Source: CAD feature listing. Evaluate the final solid. Frame: model axes, mm. A direction names the side the tool comes from. Round coordinates to 2 decimals unless told otherwise and drop trailing zeros. Loops run counter-clockwise (first coordinate to the right, second up) from the corner with the lowest first, then second, coordinate; pieces in that order, holes last.
(1) Material intervals for probe 1 along X at (y, z) = (0, 5); probe 2 along X at (y, z) = (16, 2) (3 decimals); probe 3 along Z at (x, y) = (11.25, -2), sorted ascending.
(2) First-contact query: pin 1 Ø5.5 at (x, y) = (7.94, 0) entering from +Z (3 decimals); pin 2 Ø5 at (y, z) = (-10.1, 10.1) entering from -X; pin 3 Ø2 at (x, y) = (2, 13) entering from +Z; pin 4 Ø6 at (x, y) = (1.5, 14.5) entering from +Z. Flat tips, straight axial feed; report the tip coordinate or a pass-through.
(3) Section D-D, the plane z = 5. Return the cut outline in (x, y) (1 decimal), plus the area to 3 significant figures.
(4) Section B-B, the plane x = 2. Return the cut outline in (y, z).
(5) Section A-A, the plane z = 11. Return the cut outline in (x, y) (3 decimals), plus the area to 3 significant figures.
(6) Mould query, pull axis Z, two halves, no side actions, for faces 3 (the cylindrical face through (1.565, -8.319, 8.735)), 4 (the cylindrical face through (9.663, 0.076, 6.049)), 5 (the cylindrical face through (1.565, 11.887, 8.735)), 6 (the cylindrical face through (7.87, -2.06, -9.3)). Classes: pulls with the +Z half, pulls with the -Z half, needs draft (parallel to the pull), parting line crosses it, or undercut.
(7) Section C-C, the plane y = -4. Return the cut outline in (x, z) (3 decimals).
(8) Set-up query: faces 1 (the cylindrical face through (1.57, -15.12, -11.59)), 2 (the flat face through (3.175, 4, 9)). Return all of +Z, -Z, +X, -X, +Y, -Y with unobstructed straight access to the full face (end or side cutting, diameter ignored); none if empty.
```python
from build123d import *

# Parameters (mm, degrees)
F0_R     = 19.05
F1_DEPTH = 3.175
F2_R     = 9.525
F3_DEPTH = 9.525
F5_D     = 6.35
F5_DEPTH = 9.525
F5_TIP   = 1.9077324654
F8_D     = 3.4544
F8_DEPTH = 9.525
F8_START = 0.1579085
F8_TIP   = 1.0378064612
F10_D    = 4.4958


with BuildPart() as f1:
    # F0 (on Right) → F1 (new body)
    with BuildSketch(Plane.YZ):
        Circle(F0_R)
    extrude(amount=F1_DEPTH)

    # F2 (on face) → F3 (join)
    with BuildSketch(Plane.YZ.offset(3.175)):
        Circle(F2_R)
    extrude(amount=F3_DEPTH)

    # F5
    with Locations(Plane.YZ.offset(12.7)):
        with Locations((0, 0)):
            Hole(F5_D / 2, depth=F5_DEPTH)
            with Locations((0, 0, -(F5_DEPTH + F5_TIP / 2))):  # 118° drill point
                Cone(0, F5_D / 2, F5_TIP, mode=Mode.SUBTRACT)

    # F8
    # its depths count from where the whole tool has entered the part; down to there all is cleared
    with Locations(Plane.XY.offset(9.525).offset(-F8_START)):
        with Locations((7.9375, 0)):
            Hole(F8_D / 2, depth=F8_DEPTH)
            with Locations((0, 0, -(F8_DEPTH + F8_TIP / 2))):  # 118° drill point
                Cone(0, F8_D / 2, F8_TIP, mode=Mode.SUBTRACT)

    # F10 (through all)
    with Locations(Plane.YZ.offset(3.175)):
        with Locations((-10.1027881362, 10.1027881362), (10.1027881362, 10.1027881362), (10.1027881362, -10.1027881362), (-10.1027881362, -10.1027881362)):
            Hole(F10_D / 2)


solid = f1.part
```
Output values:
1. probe 1: x = 0 to 6.21, 9.66 to 12.7
1. probe 2: x = 0 to 3.175
1. probe 3: z = -9.31 to -2.47, 2.47 to 9.31
2. pin 1: stops at z = 9.525
2. pin 2: stops at x = 0
2. pin 3: stops at z = 14.8
2. pin 4: stops at z = 15.19
3. outline: (0, -18.4) - (3.2, -18.4) - (3.2, -8.1) - (12.7, -8.1) - (12.7, 8.1) - (3.2, 8.1) - (3.2, 18.4) - (0, 18.4) - close; hole circle Ø3.5 at (7.9, 0)
3. area: 262 mm2
4. outline: circle Ø38.1 at (0, 0); hole circle Ø4.5 at (-10.1, -10.1); hole circle Ø4.5 at (-10.1, 10.1); hole circle Ø2.44 at (0, 0); hole circle Ø4.5 at (10.1, -10.1); hole circle Ø4.5 at (10.1, 10.1)
5. outline: (0, -15.553) - (3.175, -15.553) - (3.175, -12.164) - (0, -12.164) - close; (0, -8.042) - (3.175, -8.042) - (3.175, 8.042) - (0, 8.042) - close; (0, 12.164) - (3.175, 12.164) - (3.175, 15.553) - (0, 15.553) - close
5. area: 72.6 mm2
6. face 3: undercut
6. face 4: needs draft
6. face 5: undercut
6. face 6: parting line crosses it
7. outline: (0, -18.625) - (3.175, -18.625) - (3.175, -8.644) - (12.7, -8.644) - (12.7, 8.644) - (3.175, 8.644) - (3.175, 18.625) - (0, 18.625) - close
8. face 1: +X, -X
8. face 2: +X
